Answer from the drawing. Dimensions are ordinates in mm from the lowest x, y and z of the part. A direction names the side the tool comes from. Coordinates: 2 decimals unless noted, no trailing zeros. Loops run counter-clockwise (first coordinate to the right, second up) from the corner with the lowest first, then second, coordinate; pieces in that order, holes last. Notation, with made-up numbers: (7, 75.25) -> (28, 75.25) arc R20 ccw to (28, 79.25) -> close; hole circle Ø11 at (66.5, -22). An arc over 180 degrees is marked (long way). Use a Markdown table: item, result.
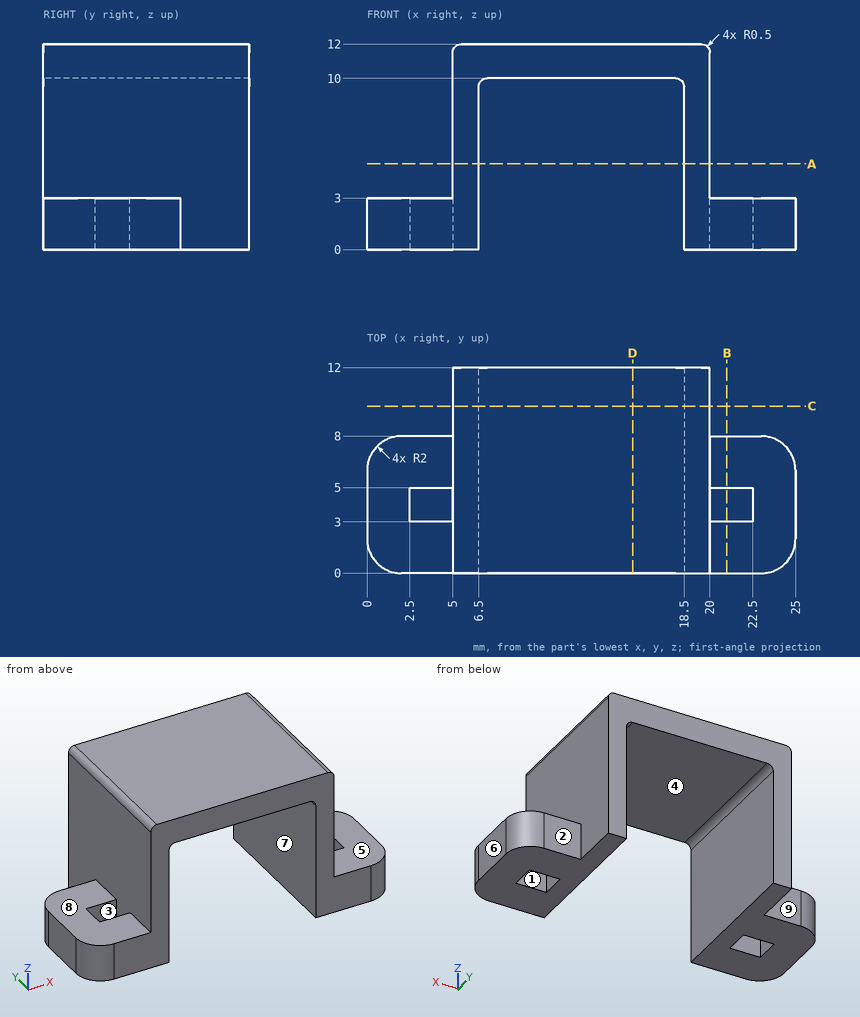
Q1. Given pin 1 Ø5.5 at (x, y) = (12, 7) entering from -Z; pin 2 Ø5 at (y, z) = (9, 3) entering from -X; pin 3 Ø0.9 at (x, z) = (3, 1.5) entering from +Y, each flat-ended and moving along its own axis, determine where each tip first touches the part or whether it passes through.
Solved:
| item | result |
|---|---|
| pin 1 | z = 10 |
| pin 2 | x = 0.06 |
| pin 3 | y = 8 |
Q2. Consider line 1 (X direction, y = 9.25, z = 7.25); line 2 (Z direction, x = 8, y = 1.5); line 3 (X direction, y = 7.25, z = 0.5). Determine where each line is inside the solid, lowest interval first. Write a range as [from, to].
Solved:
| item | result |
|---|---|
| line 1 | [5, 6.5], [18.5, 20] |
| line 2 | [10, 12] |
| line 3 | [0.44, 6.5], [18.5, 24.56] |
Q3. Determine the mould class of the marked faces 1, 2, 3 and 4 for opening direction Y: pulls with the +Y half, pulls with the -Y half, needs draft (parallel to the pull), parting line crosses it, or undercut.
Solved:
| item | result |
|---|---|
| face 1 | undercut |
| face 2 | pulls with the +Y half |
| face 3 | undercut |
| face 4 | needs draft |
Q4. Section A-A on z = 5 is taken. Determine the outline of the cut face in (x, y), and give its area (3 significant figures).
Solved:
| item | result |
|---|---|
| outline | (5, 0) -> (6.5, 0) -> (6.5, 12) -> (5, 12) -> close; (18.5, 0) -> (20, 0) -> (20, 12) -> (18.5, 12) -> close |
| area | 36.0 mm² |
Q5. Section C-C on y = 9.75 is taken. Determine the outline of the cut face in (x, z), and give its area (3 significant figures).
Solved:
| item | result |
|---|---|
| outline | (5, 0) -> (6.5, 0) -> (6.5, 9.5) arc R0.5 cw to (7, 10) -> (18, 10) arc R0.5 cw to (18.5, 9.5) -> (18.5, 0) -> (20, 0) -> (20, 11.5) arc R0.5 ccw to (19.5, 12) -> (5.5, 12) arc R0.5 ccw to (5, 11.5) -> close |
| area | 60.0 mm² |
Q6. For the marked faces 5, 6, 7, 8 and 9, determine the directions among +Z, -Z, +X, -X, +Y, -Y from which every point of the face is accessible in a straight line to the end or side of a thin tool.
Solved:
| item | result |
|---|---|
| face 5 | +Z, +X, +Y, -Y |
| face 6 | +Z, -Z, +X, +Y, -Y |
| face 7 | -Z, +Y, -Y |
| face 8 | +Z, -X, +Y, -Y |
| face 9 | +Z, -Z, -X, +Y |
Q7. Section D-D on x = 15.5 is taken. Determine the outline of the cut face in (y, z).
Solved:
| item | result |
|---|---|
| outline | (0, 10) -> (12, 10) -> (12, 12) -> (0, 12) -> close |
Q8. Section B-B on x = 21 is taken. Determine the outline of the cut face in (y, z).
Solved:
| item | result |
|---|---|
| outline | (0, 0) -> (3, 0) -> (3, 3) -> (0, 3) -> close; (5, 0) -> (8, 0) -> (8, 3) -> (5, 3) -> close |
